Geometry check sheet. Reference: drawing and pictorial views, mm from the part's lowest x, y, z. Give positions to 0.01 mm unless a question says otherwise; leave off trailing zeros. Write each loop counter-clockwise with the first axis right and the second up, starting at its lowest first coordinate (ties: lowest second). Pieces come first, ordered by that corner, then holes. Notation, with made-up numbers: M 7,46 L 65,46 A25 ccw 65,83 Z; hole C 35.25,-31 d11. An arc over 180 degrees is marked long. Answer as a JSON object with one key per item and string values.
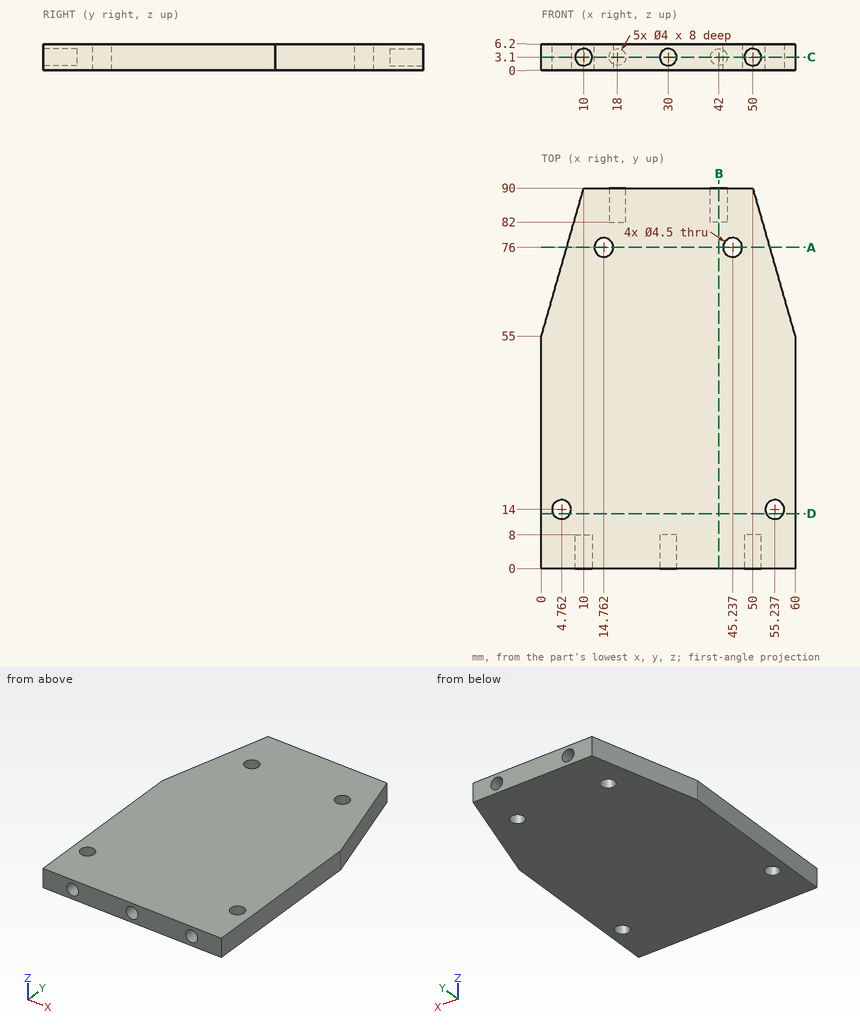
1) Section check B-B on x = 42. Record the boundary of the cut face in (y, z), and give its area (3 significant figures).
Completed:
{"outline": "M 0,0 L 90,0 L 90,1.1 L 82,1.1 L 82,5.1 L 90,5.1 L 90,6.2 L 0,6.2 Z", "area": "526 mm2"}
2) Section check C-C on z = 3.1. Count the separate pieces of the cut face and the enclosed holes in it, and give its area (3 significant figures).
Completed:
{"separate pieces": "1", "enclosed holes": "4", "area": "4,830 mm2"}
3) Section check A-A on y = 76. Record the boundary of the cut face in (x, z).
Completed:
{"outline": "M 6,0 L 12.51,0 L 12.51,6.2 L 6,6.2 Z; M 17.01,0 L 42.99,0 L 42.99,6.2 L 17.01,6.2 Z; M 47.49,0 L 54,0 L 54,6.2 L 47.49,6.2 Z"}
4) Thickness scan on L1, parallel to Y at x = 45, z = 1.25; L2, parallel to Z at x = 10, y = 2.5; L3, parallel to X at y = 74.5, z = 0.5 (1 decimal). Record the ranges inside material, lowest first.
Completed:
{"L1": "y = 0 to 73.76, 78.24 to 90", "L2": "z = 0 to 1.1, 5.1 to 6.2", "L3": "x = 5.6 to 13.1, 16.4 to 43.6, 46.9 to 54.4"}
5) Section check D-D on y = 13. Record the boundary of the cut face in (x, z), and give its area (3 significant figures).
Completed:
{"outline": "M 0,0 L 2.75,0 L 2.75,6.2 L 0,6.2 Z; M 6.78,0 L 53.22,0 L 53.22,6.2 L 6.78,6.2 Z; M 57.25,0 L 60,0 L 60,6.2 L 57.25,6.2 Z", "area": "322 mm2"}
6) Go/stop test with flat-tipped pins: pin 1 (1.2 mm diameter, centred on x = 42.5, z = 4, fed in from +Y); pin 2 (1 mm diameter, centred on x = 13, y = 80.5, fed in from -Z); pin 3 (2 mm diameter, centred on x = 30.5, z = 2.5, fed in from -Y). Record where each tip stops, or that it passes through.
Completed:
{"pin 1": "stops at y = 82", "pin 2": "stops at z = 0", "pin 3": "stops at y = 8"}
